from build123d import *

# Parameters (mm, degrees)
F0_R          = 17
F1_DEPTH      = 60
F2_R          = 15
F3_DEPTH      = 40
F4_R          = 15
F5_DEPTH      = 15
F6_W          = 2.5
F6_H          = 10
F7_DEPTH      = 18
F7_DEPTH_BACK = 18
F8_W          = 17
F8_H          = 2.5
F10_ANGLE     = 90
F11_W         = 17
F11_H         = 2.5
F12_ANGLE     = 90


with BuildPart() as f1:
    # F0 (on Top) → F1 (new body)
    with BuildSketch(Plane.XY):
        Circle(F0_R)
    extrude(amount=F1_DEPTH)

    # F2 (on face) → F3 (cut)
    with BuildSketch(Plane.XY.offset(60)):
        Circle(F2_R)
    extrude(amount=-F3_DEPTH, mode=Mode.SUBTRACT)

    # F4 (on face) → F5 (cut)
    with BuildSketch(Plane(origin=(0, 0, 0), x_dir=(1, 0, 0), z_dir=(0, 0, -1))):
        Circle(F4_R)
    extrude(amount=-F5_DEPTH, mode=Mode.SUBTRACT)

    # F6 (on Right) → F7 (cut, two sides)
    with BuildSketch(Plane.YZ) as f7_sk:
        with Locations((0, 5)):
            Rectangle(F6_W, F6_H)
    extrude(amount=F7_DEPTH, mode=Mode.SUBTRACT)
    extrude(f7_sk.sketch, amount=-F7_DEPTH_BACK, mode=Mode.SUBTRACT)

    # F8 (on Front) → F10 (revolve, cut)
    with BuildSketch(Plane.XZ):
        with Locations((-8.5, 8.75)):
            Rectangle(F8_W, F8_H)
    revolve(axis=Axis((0, 0, 15.6492851675), (0, 0, -1)), revolution_arc=F10_ANGLE, mode=Mode.SUBTRACT)

    # F11 (on Front) → F12 (revolve, cut)
    with BuildSketch(Plane.XZ):
        with Locations((8.5, 8.75)):
            Rectangle(F11_W, F11_H)
    revolve(axis=Axis((0, 0, 6.5289476479), (0, 0, -1)), revolution_arc=F12_ANGLE, mode=Mode.SUBTRACT)

    # F13 (on Front) → F14 (revolve, cut)
    with BuildSketch(Plane.XZ):
        with BuildLine():
            Line((-2.4, 15), (0, 15))
            Line((0, 15), (0, 20))
            Line((0, 20), (-2.4, 20))
            Line((-2.4, 20), (-2.4, 18.6))
            Line((-2.4, 18.6), (-3.5, 18.6))
            ThreePointArc((-3.5, 18.6), (-4.6, 17.5), (-3.5, 16.4))
            Line((-3.5, 16.4), (-2.4, 16.4))
            Line((-2.4, 16.4), (-2.4, 15))
        make_face()
    revolve(axis=Axis((0, 0, 17.5), (0, 0, 1)), mode=Mode.SUBTRACT)


solid = f1.part
Geometry: final body of the model. Coordinates: model frame, mm. A direction names the side the tool comes from. Coordinates: 2 decimals unless noted, no trailing zeros. Order: outer loops, then holes, each group sorted by start corner. A loop starts at its lowest first (then second) coordinate and runs counter-clockwise, first axis right, second up.
(1) Section query B-B (x = -13.5). Return the cut outline in (y, z), plus the area to 3 significant figures.
(2) Draft query along Z for faces 1 (the face through (0, -16, 0)), 2 (the face through (0, -16, 9)), 3 (the face through (-1.29, -2.024, 19.29)), 4 (the face through (-11, 11, 10)). Return one class per face: pulls with the +Z half, pulls with the -Z half, needs draft (parallel to the pull), parting line crosses it, or undercut.
(3) Section query A-A (y = 0). Return the cut outline in (x, z), plus the area to 3 significant figures.
(4) Section query D-D (y = 14). Return the cut outline in (x, z), plus the area to 3 significant figures.
(5) Material intervals for probe 1 along Y at (x, z) = (0, 11.75); probe 2 along Y at (x, z) = (0, 15.55); probe 3 along Z at (x, y) = (-9, 13), sorted ascending.
(6) Access query for faces 5 (the face through (3, 0, 20)), 6 (the face through (13.856, 5.745, 7.395)), 7 (the face through (-11, 11, 7.5)), 8 (the face through (11, -11, 10)), 9 (the face through (-16, -1.25, 5)). Directions: +Z, -Z, +X, -X, +Y, -Y. A direction counts if a zero-diameter tool reaches every point of the face in a straight line with its end or side. Return the directions, or none.
(7) First-contact query: pin 1 (8 mm diameter, centred on x = 13.5, z = 49.5, fed in from -Y); pin 2 (1.5 mm diameter, centred on x = -1.5, z = 28, fed in from +Y); pin 3 (12 mm diameter, centred on y = 9, z = 33.5, fed in from +X). Flat tips, straight axial feed; report the tip coordinate or a pass-through.
(8) Section query C-C (z = 51.5). Return the cut outline in (x, y), plus the area to 3 significant figures.
Solution:
1. outline: (-10.33, 0) - (-6.54, 0) - (-6.54, 15) - (6.54, 15) - (6.54, 10) - (10.33, 10) - (10.33, 60) - (6.54, 60) - (6.54, 20) - (-6.54, 20) - (-6.54, 60) - (-10.33, 60) - close; (6.54, 0) - (10.33, 0) - (10.33, 7.5) - (6.54, 7.5) - close
1. area: 511 mm2
2. face 1: pulls with the -Z half
2. face 2: undercut
2. face 3: needs draft
2. face 4: undercut
3. outline: (-17, 10) - (-15, 10) - (-15, 15) - (-2.4, 15) - (-2.4, 16.4) - (-3.5, 16.4) arc R1.1 cw to (-3.5, 18.6) - (-2.4, 18.6) - (-2.4, 20) - (-15, 20) - (-15, 60) - (-17, 60) - close; (2.4, 15) - (15, 15) - (15, 10) - (17, 10) - (17, 60) - (15, 60) - (15, 20) - (2.4, 20) - (2.4, 18.6) - (3.5, 18.6) arc R1.1 cw to (3.5, 16.4) - (2.4, 16.4) - close
3. area: 317 mm2
4. outline: (-9.64, 0) - (-5.39, 0) - (-5.39, 7.5) - (-9.64, 7.5) - close; (-9.64, 10) - (-5.39, 10) - (-5.39, 15) - (5.39, 15) - (5.39, 0) - (9.64, 0) - (9.64, 60) - (5.39, 60) - (5.39, 20) - (-5.39, 20) - (-5.39, 60) - (-9.64, 60) - close
4. area: 554 mm2
5. probe 1: y = -17 to -15, 15 to 17
5. probe 2: y = -17 to -2.4, 2.4 to 17
5. probe 3: z = 0 to 7.5, 10 to 60
6. face 5: +Z
6. face 6: -Z
6. face 7: -X, +Y
6. face 8: +X, -Y
6. face 9: -Z, +X, -X
7. pin 1: stops at y = -14.1
7. pin 2: stops at y = 16.98
7. pin 3: stops at x = 16.73
8. outline: circle Ø34 at (0, 0); hole circle Ø30 at (0, 0)
8. area: 201 mm2
